Here's how the part is built. I have some questions about the finished solid (model axes, mm). A direction names the side the tool comes from. Coordinates: 2 decimals unless noted, no trailing zeros. Write each loop counter-clockwise with the first axis right and the second up, starting at its lowest first coordinate (ties: lowest second). Pieces come first, ordered by that corner, then holes.
```python
from build123d import *

# Parameters (mm, degrees)
ESQUISSE1_W             = 45
ESQUISSE1_H             = 135
ESQUISSE1_R             = 1.25
BOSS_EXTRU_1_DEPTH      = 6
ENL_V_MAT_EXTRU_1_DEPTH = 143.428929646


with BuildPart() as part:
    # Esquisse1 → Boss.-Extru.1 (new body)
    with BuildSketch(Plane.XY):
        with Locations((22.5, 67.5)):
            Rectangle(ESQUISSE1_W, ESQUISSE1_H)
        with Locations((8, 5)):
            Circle(ESQUISSE1_R, mode=Mode.SUBTRACT)
        with Locations((8, 15)):
            Circle(ESQUISSE1_R, mode=Mode.SUBTRACT)
        with Locations(Location((8, 120, 0), (0, 0, 180))):
            Circle(ESQUISSE1_R, mode=Mode.SUBTRACT)
        with Locations(Location((8, 130, 0), (0, 0, 180))):
            Circle(ESQUISSE1_R, mode=Mode.SUBTRACT)
    extrude(amount=BOSS_EXTRU_1_DEPTH)

    # Esquisse2 → Enlèv. mat.-Extru.1 (cut, through all)
    with BuildSketch(Plane(origin=(0, 0, 0), x_dir=(-1, 0, 0), z_dir=(0, 0, -1))):
        with BuildLine():
            Line((0, 25.080128411), (0, 113.33030278))
            Line((0, 113.33030278), (-15, 113.33030278))
            Line((-15, 113.33030278), (-15, 68.33030278))
            ThreePointArc((-15, 68.33030278), (-21.619788224, 41.80819896), (0, 25.080128411))
        make_face()
    extrude(amount=-ENL_V_MAT_EXTRU_1_DEPTH, mode=Mode.SUBTRACT)


solid = part.part
```
1) I need wall thicknesses on probe 1 along X at (y, z) = (120, 4); probe 2 along Y at (x, z) = (8, 4.75); probe 3 along Y at (x, z) = (8.5, 2.6). Which ranges of each line are inside material? Lowest first, please.
Values follow:
probe 1: x = 0 to 6.75, 9.25 to 45
probe 2: y = 0 to 3.75, 6.25 to 13.75, 16.25 to 27.09, 113.33 to 118.75, 121.25 to 128.75, 131.25 to 135
probe 3: y = 0 to 3.85, 6.15 to 13.85, 16.15 to 27.31, 113.33 to 118.85, 121.15 to 128.85, 131.15 to 135
2) We'd pull the mould along X, two halves only. Please class faces 3 (the face through (21.75, 42.19, 2.96)), 4 (the face through (22, 135, 3)), 5 (the face through (7.079, 15.845, 2.958)): pulls with the +X half, pulls with the -X half, needs draft (parallel to the pull), parting line crosses it, or undercut.
Values follow:
face 3: pulls with the -X half
face 4: needs draft
face 5: undercut
3) Imagine slicing it at C-C on x = 8. Please give me the cut outline in (y, z), then the cut area to 3 significant figures.
Values follow:
outline: (0, 0) - (3.75, 0) - (3.75, 6) - (0, 6) - close; (6.25, 0) - (13.75, 0) - (13.75, 6) - (6.25, 6) - close; (16.25, 0) - (27.09, 0) - (27.09, 6) - (16.25, 6) - close; (113.33, 0) - (118.75, 0) - (118.75, 6) - (113.33, 6) - close; (121.25, 0) - (128.75, 0) - (128.75, 6) - (121.25, 6) - close; (131.25, 0) - (135, 0) - (135, 6) - (131.25, 6) - close
area: 233 mm2
4) Imagine slicing it at A-A on y = 130. Please give me the cut outline in (x, z), then the cut area to 3 significant figures.
Values follow:
outline: (0, 0) - (6.75, 0) - (6.75, 6) - (0, 6) - close; (9.25, 0) - (45, 0) - (45, 6) - (9.25, 6) - close
area: 255 mm2
5) On a 3-axis mill with a long thin cutter (end or side, diameter ignored), from which of +Z, -Z, +X, -X, +Y, -Y can I reach the whole of each face in a straight line? I mean faces 1 (the face through (22, 0, 3)), 2 (the face through (15, 91, 3)). Say none if no direction works.
Values follow:
face 1: +Z, -Z, +X, -X, -Y
face 2: +Z, -Z, -X
6) Will these pins go through, and if not, where does the flat tip stop? pin 1 (1.8 mm diameter, centred on x = 10, z = 2, fed in from -Y); pin 2 (2 mm diameter, centred on x = 8, y = 120, fed in from +Z).
Values follow:
pin 1: stops at y = 0
pin 2: passes through
7) Imagine slicing it at B-B on z = 5.1. Please give me the cut outline in (x, y), then the cut area to 3 significant figures.
Values follow:
outline: (0, 0) - (45, 0) - (45, 135) - (0, 135) - (0, 113.33) - (15, 113.33) - (15, 68.33) arc R25 cw to (0, 25.08) - close; hole circle Ø2.5 at (8, 5); hole circle Ø2.5 at (8, 15); hole circle Ø2.5 at (8, 120); hole circle Ø2.5 at (8, 130)
area: 4,560 mm2
8) Imagine slicing it at D-D on y = 112. Please give me the cut outline in (x, z).
Values follow:
outline: (15, 0) - (45, 0) - (45, 6) - (15, 6) - close
